The listing builds one solid part. Answer for the finished solid, in the listing's coordinates (mm). A direction names the side the tool comes from. Give positions to 0.01 mm unless a question says otherwise; leave off trailing zeros. Write each loop counter-clockwise with the first axis right and the second up, starting at its lowest first coordinate (ties: lowest second). Pieces come first, ordered by that corner, then holes.
```python
from build123d import *

# Parameters (mm, degrees)
EXTRUDE_START       = 38.5
SKETCH_4_W          = 25
SKETCH_4_H          = 25
EXTRUDE_1_DEPTH     = 14.5
SKETCH_5_R          = 11.875
EXTRUDE_2_DEPTH     = 62.5
SKETCH_6_R          = 10
EXTRUDE_3_DEPTH     = 14
EXTRUDE_START_2     = 49.5
EXTRUDE_4_DEPTH     = 8
SKETCH_8_R          = 4.864
CUT_EXTRUDE_1_DEPTH = 4.994447
SKETCH_9_OUTSIDE_W  = 47.858
SKETCH_9_OUTSIDE_H  = 51.88
SKETCH_9_OUTSIDE_R  = 14.5
CUT_EXTRUDE_2_DEPTH = 77
SKETCH_11_R         = 4
CUT_EXTRUDE_3_DEPTH = 76.5
CHAMFER_1_SIZE      = 0.7
CHAMFER_2_SIZE      = 0.59728
EXTRUDE_START_3     = 13
SKETCH_12_R         = 10
EXTRUDE_5_DEPTH     = 13
CUT_EXTRUDE_START   = 1.3
SKETCH_13_R         = 10
SKETCH_13_R_2       = 9
CUT_EXTRUDE_4_DEPTH = 1.3
CHAMFER_3_SIZE      = 0.7


with BuildPart() as part:
    # 草图4 → 凸台-拉伸1 (new body)
    with BuildSketch(Plane.XY.offset(EXTRUDE_START)):
        Rectangle(SKETCH_4_W, SKETCH_4_H)
    extrude_1 = extrude(amount=-EXTRUDE_1_DEPTH)

    # 草图5 → 凸台-拉伸2 (add)
    with BuildSketch(Plane(origin=(0, 0, 24), x_dir=(-1, 0, 0), z_dir=(0, 0, -1))):
        Circle(SKETCH_5_R)
    extrude(amount=EXTRUDE_2_DEPTH)

    # 镜向1: 凸台-拉伸1 across plane
    add(extrude_1.mirror(Plane.XY))

    # 草图6 → 凸台-拉伸3 (add)
    with BuildSketch(Plane.XY.offset(38.5)):
        with Locations(Location((0, 0, 0), (0, 0, 180))):
            Circle(SKETCH_6_R)
    extrude(amount=EXTRUDE_3_DEPTH)

    # 草图7 → 凸台-拉伸4 (add)
    with BuildSketch(Plane.XY.offset(EXTRUDE_START_2)):
        Polygon((13, 7.505553499), (0, 15.011106999), (-13, 7.505553499), (-13, -7.505553499), (0, -15.011106999), (13, -7.505553499), align=None)
    extrude(amount=-EXTRUDE_4_DEPTH)

    # 草图10 → 切除-旋转1 (revolve, cut)
    with BuildSketch(Plane(origin=(0, 0, 0), x_dir=(1, 0, 0), z_dir=(0, 1, 0)), mode=Mode.PRIVATE) as cut_revolve_1_sk:
        Polygon((-13, -49.5), (-25.989909678, -49.5), (-25.989909678, -41.5), (-13, -41.5), (-23.989909678, -45.5), align=None)
    revolve(cut_revolve_1_sk.sketch.rotate(Axis((0, 0, 52.5), (0, 0, 1)), 180), axis=Axis((0, 0, 52.5), (0, 0, 1)), mode=Mode.SUBTRACT)

    # 草图8 → 切除-拉伸1 (cut)
    with BuildSketch(Plane(origin=(0, 12.5, 0), x_dir=(1, 0, 0), z_dir=(0, 1, 0))):
        with Locations(Location((0, -31, 0), (0, 0, 270))):
            Circle(SKETCH_8_R)
    cut_extrude_1 = extrude(amount=-CUT_EXTRUDE_1_DEPTH, mode=Mode.SUBTRACT)

    # 镜向2: 切除-拉伸1 across plane
    add(cut_extrude_1.mirror(Plane.XY), mode=Mode.SUBTRACT)

    # 草图9 outside → 切除-拉伸2 (cut)
    with BuildSketch(Plane.XY.offset(38.5)):
        Rectangle(SKETCH_9_OUTSIDE_W, SKETCH_9_OUTSIDE_H)
        Circle(SKETCH_9_OUTSIDE_R, mode=Mode.SUBTRACT)
    extrude(amount=-CUT_EXTRUDE_2_DEPTH, mode=Mode.SUBTRACT)

    # 草图11 → 切除-拉伸3 (cut)
    with BuildSketch(Plane.XY.offset(52.5)):
        Circle(SKETCH_11_R)
    extrude(amount=-CUT_EXTRUDE_3_DEPTH, mode=Mode.SUBTRACT)

    # 倒角1
    chamfer_1_edges = [part.edges().sort_by_distance(p)[0] for p in [
        (10, 0, 52.5),
    ]]
    chamfer(chamfer_1_edges, length=CHAMFER_1_SIZE)

    # 倒角2
    chamfer_2_edges = [part.edges().sort_by_distance(p)[0] for p in [
        (0, 12.5, 26.136),
        (0, 12.5, -26.136),
    ]]
    chamfer(chamfer_2_edges, length=CHAMFER_2_SIZE)

    # 草图12 → 凸台-拉伸5 (add)
    with BuildSketch(Plane(origin=(0, 0, -38.5), x_dir=(-1, 0, 0), z_dir=(0, 0, -1)).offset(EXTRUDE_START_3)):
        Circle(SKETCH_12_R)
    extrude(amount=-EXTRUDE_5_DEPTH)

    # 草图13 → 切除-拉伸4 (cut)
    with BuildSketch(Plane(origin=(0, 0, -38.5), x_dir=(-1, 0, 0), z_dir=(0, 0, -1)).offset(CUT_EXTRUDE_START)):
        Circle(SKETCH_13_R)
        Circle(SKETCH_13_R_2, mode=Mode.SUBTRACT)
    extrude(amount=-CUT_EXTRUDE_4_DEPTH, mode=Mode.SUBTRACT)

    # 倒角3
    chamfer_3_edges = [part.edges().sort_by_distance(p)[0] for p in [
        (10, 0, -51.5),
    ]]
    chamfer(chamfer_3_edges, length=CHAMFER_3_SIZE)


solid = part.part
```
Item 1: A cutting plane is placed at D-D, the plane z = -18. Give the vertices of the cut face in (x, y) (3 decimals), plus the area to 3 significant figures.
Conclusion:
outline: circle Ø23.75 at (0, 0); hole circle Ø8 at (0, 0)
area: 393 mm2
Item 2: A cutting plane is placed at B-B, the plane z = -31. Give the vertices of the cut face in (x, y), plus the area to 3 significant figures.
Conclusion:
outline: (-12.5, -7.35) arc R14.5 ccw to (-7.35, -12.5) - (7.35, -12.5) arc R14.5 ccw to (12.5, -7.35) - (12.5, 7.35) arc R14.5 ccw to (7.35, 12.5) - (5.46, 12.5) - (4.86, 11.9) - (4.86, 7.51) - (-4.86, 7.51) - (-4.86, 11.9) - (-5.46, 12.5) - (-7.35, 12.5) arc R14.5 ccw to (-12.5, 7.35) - close
area: 532 mm2
Item 3: Each of these flat-tipped pins is pushed along its axis until it touches: P1, Ø10, axis at x = 8, z = -21.5, coming from the -Y side; P2, Ø4, axis at y = -1, z = -37, coming from the +X side; P3, Ø4, axis at y = -4, z = -13, coming from the -X side; P4, Ø4, axis at x = 2, y = 1, coming from the +Z side. Where does it stop, or does it pass through?
Conclusion:
P1: stops at y = -12.5
P2: stops at x = 12.5
P3: stops at x = -11.71
P4: stops at z = 52.5
Item 4: Consider probe 1 along Y at (x, z) = (0, -7) (3 decimals); probe 2 along Z at (x, y) = (8, 8.5); probe 3 along Z at (x, y) = (7.5, -5.5). Determine where each line is inside the solid, lowest interval first.
Conclusion:
probe 1: y = -11.875 to -4, 4 to 11.875
probe 2: z = -38.5 to 38.5, 41.5 to 49.5
probe 3: z = -51.5 to -39.8, -38.5 to 52.5
Item 5: Which of the six approach directions +Z, -Z, +X, -X, +Y, -Y give full straight-line access (tool end or side, diameter ignored) to faces 4 (the face through (-11.7, -6.72, 41.68)), 5 (the face through (-3, 9, -38.5)), 6 (the face through (2.17, -9.76, -45.38)), 7 (the face through (0, 7.506, -31))?
Conclusion:
face 4: -X, -Y
face 5: none
face 6: -Z
face 7: +Y
Item 6: Determine the mould class of faces 1 (the face through (10, 0, 51)), 2 (the face through (11.657, -6.768, 49.325)), 3 (the face through (9, 2, -39.8)) for opening direction Z: pulls with the +Z half, pulls with the -Z half, needs draft (parallel to the pull), parting line crosses it, or undercut.
Conclusion:
face 1: needs draft
face 2: pulls with the +Z half
face 3: undercut
Item 7: A cutting plane is placed at C-C, the plane z = 31. Give the vertices of the cut face in (x, y), plus the area to 3 significant figures.
Conclusion:
outline: (-12.5, -7.35) arc R14.5 ccw to (-7.35, -12.5) - (7.35, -12.5) arc R14.5 ccw to (12.5, -7.35) - (12.5, 7.35) arc R14.5 ccw to (7.35, 12.5) - (5.46, 12.5) - (4.86, 11.9) - (4.86, 7.51) - (-4.86, 7.51) - (-4.86, 11.9) - (-5.46, 12.5) - (-7.35, 12.5) arc R14.5 ccw to (-12.5, 7.35) - close; hole circle Ø8 at (0, 0)
area: 482 mm2
Item 8: A cutting plane is placed at A-A, the plane z = 45. Give the vertices of the cut face in (x, y), plus the area to 3 significant figures.
Conclusion:
outline: (-13, -7.51) - (0, -15.01) - (13, -7.51) - (13, 7.51) - (0, 15.01) - (-13, 7.51) - close; hole circle Ø8 at (0, 0)
area: 535 mm2
